Here's how the part is built. I have some questions about the finished solid (model axes, mm). A direction names the side the tool comes from. Give positions to 0.01 mm unless a question says otherwise; leave off trailing zeros. Write each loop counter-clockwise with the first axis right and the second up, starting at its lowest first coordinate (ties: lowest second). Pieces come first, ordered by that corner, then holes. Notation, with made-up numbers: (-8.75, -9) -> (45.25, -9) arc R23 ccw to (45.25, 19) -> close; hole circle Ø10 at (38, -7). An arc over 180 degrees is marked (long way). Use one line per item in the form item = value.
```python
from build123d import *

# Parameters (mm, degrees)
SKETCH1_W           = 30
SKETCH1_H           = 25
BOSS_EXTRUDE1_DEPTH = 20
SKETCH2_W           = 15
SKETCH2_H           = 25
CUT_EXTRUDE1_DEPTH  = 10
CUT_EXTRUDE2_DEPTH  = 20
SKETCH4_W           = 10
SKETCH4_H           = 15
CUT_EXTRUDE3_DEPTH  = 15


with BuildPart() as part:
    # Sketch1 → Boss-Extrude1 (new body)
    with BuildSketch(Plane.XY):
        with Locations((15, 12.5)):
            Rectangle(SKETCH1_W, SKETCH1_H)
    extrude(amount=BOSS_EXTRUDE1_DEPTH)

    # Sketch2 → Cut-Extrude1 (cut)
    with BuildSketch(Plane.XY.offset(20)):
        with Locations((7.5, 12.5)):
            Rectangle(SKETCH2_W, SKETCH2_H)
    extrude(amount=-CUT_EXTRUDE1_DEPTH, mode=Mode.SUBTRACT)

    # Sketch3 → Cut-Extrude2 (cut)
    with BuildSketch(Plane.ZY.offset(-15)):
        Polygon((15, 25), (20, 15), (20, 25), align=None)
    extrude(amount=-CUT_EXTRUDE2_DEPTH, mode=Mode.SUBTRACT)

    # Sketch4 → Cut-Extrude3 (cut)
    with BuildSketch(Plane.ZY):
        with Locations((5, 7.5)):
            Rectangle(SKETCH4_W, SKETCH4_H)
    extrude(amount=-CUT_EXTRUDE3_DEPTH, mode=Mode.SUBTRACT)


solid = part.part
```
Q1. Which directions (+Z, -Z, +X, -X, +Y, -Y) give clear straight access to the entire face, cutting with the end or side of a thin tool? Please do faces 1 (the face through (0, 20, 5)), 2 (the face through (7, 15, 5)), 3 (the face through (7, 20, 10)).
Result set:
face_1 = +Z, -Z, -X, +Y, -Y
face_2 = +Z, -Z, -X, -Y
face_3 = +Z, -X, +Y, -Y
Q2. I want a section at A-A, the plane y = 20. Write out the boundary of the cut face in (x, z).
Result set:
outline = (0, 0) -> (30, 0) -> (30, 17.5) -> (15, 17.5) -> (15, 10) -> (0, 10) -> close
Q3. I want a section at B-B, the plane z = 8.5. Write out the boundary of the cut face in (x, y).
Result set:
outline = (0, 15) -> (15, 15) -> (15, 0) -> (30, 0) -> (30, 25) -> (0, 25) -> close
Q4. I want a section at D-D, the plane z = 18.5. Write out the boundary of the cut face in (x, y).
Result set:
outline = (15, 0) -> (30, 0) -> (30, 18) -> (15, 18) -> close
Q5. Will these pins go through, and if not, where does the flat tip stop? pin 1 Ø8 at (x, y) = (8, 19.5) entering from +Z; pin 2 Ø11 at (x, z) = (9, 5.5) entering from -Y.
Result set:
pin_1 = 10
pin_2 = 15
Q6. I want a section at C-C, the plane x = 26. Write out the boundary of the cut face in (y, z).
Result set:
outline = (0, 0) -> (25, 0) -> (25, 15) -> (15, 20) -> (0, 20) -> close
Q7. If I drill on line 1 along X through (y, z) = (4.25, 7.5); line 2 along Z through (x, y) = (2.75, 15.75); line 3 along Z through (x, y) = (25.75, 20.5), over which ranges is the centre line in solid material (lowest first)? Write a range as from..to.
Result set:
line_1 = 15..30
line_2 = 0..10
line_3 = 0..17.25
